```python
from build123d import *

# Parameters (mm, degrees)
SKETCH1_W              = 25.4
SKETCH1_H              = 27.78125
BOSS_EXTRUDE1_DEPTH    = 2.38125
SKETCH2_W              = 25.4
SKETCH2_H              = 2.38125
BOSS_EXTRUDE2_DEPTH    = 25.4
CONVERT_SOLID2_START   = -12.7
CONVERT_SOLID2_DEPTH   = 25.4
CONVERT_SOLID2_2_DEPTH = 25.4
FILLET1_R              = 2.54
SKETCH9_R              = 2.54
CUT_EXTRUDE1_DEPTH     = 2.38125


# Read off the part's stored shape, not the designer's step: Convert-Solid2
with BuildPart() as part:
    # Sketch1 → Boss-Extrude1 (new body)
    with BuildSketch(Plane(origin=(0, 0, 0), x_dir=(1, 0, 0), z_dir=(0, 1, 0))):
        Rectangle(SKETCH1_W, SKETCH1_H)
    extrude(amount=BOSS_EXTRUDE1_DEPTH)

    # Sketch2 → Boss-Extrude2 (add)
    with BuildSketch(Plane(origin=(0, 2.38125, 0), x_dir=(1, 0, 0), z_dir=(0, 1, 0))):
        with Locations((0, 12.7)):
            Rectangle(SKETCH2_W, SKETCH2_H)
    extrude(amount=BOSS_EXTRUDE2_DEPTH)

    # Convert-Solid2 outline → Convert-Solid2 (cut)
    with BuildSketch(Plane.YZ.offset(CONVERT_SOLID2_START)):
        with BuildLine():
            Line((0, -13.890625), (7.14375, -13.890625))
            ThreePointArc((7.14375, -13.890625), (2.092355932, -11.798269068), (0, -6.746875))
            Line((0, -6.746875), (0, -13.890625))
        make_face()
    extrude(amount=CONVERT_SOLID2_DEPTH, mode=Mode.SUBTRACT)

    # Convert-Solid2 2 outline → Convert-Solid2 2 (add)
    with BuildSketch(Plane.YZ.offset(CONVERT_SOLID2_START)):
        with BuildLine():
            Line((2.38125, -11.509375), (7.14375, -11.509375))
            ThreePointArc((7.14375, -11.509375), (3.776153955, -10.114471045), (2.38125, -6.746875))
            Line((2.38125, -6.746875), (2.38125, -11.509375))
        make_face()
    extrude(amount=CONVERT_SOLID2_2_DEPTH)

    # Fillet1
    fillet1_edges = [part.edges().sort_by_distance(p)[0] for p in [
        (-12.7, 1.190625, 13.890625),
        (12.7, 1.190625, 13.890625),
        (-12.7, 27.78125, -12.7),
        (12.7, 27.78125, -12.7),
    ]]
    fillet(fillet1_edges, radius=FILLET1_R)

    # Sketch9 → Cut-Extrude1 (cut)
    with BuildSketch(Plane(origin=(0, 2.38125, 0), x_dir=(1, 0, 0), z_dir=(0, 1, 0))):
        with Locations(Location((6.35, -7.540625, 0), (0, 0, 270))):
            Circle(SKETCH9_R)
        with Locations(Location((-6.35, -7.540625, 0), (0, 0, 270))):
            Circle(SKETCH9_R)
    extrude(amount=-CUT_EXTRUDE1_DEPTH, mode=Mode.SUBTRACT)


solid = part.part
```
Model file for the job. Use its own axes, mm. A direction names the side the tool comes from. Round coordinates to 2 decimals unless told otherwise and drop trailing zeros. Write each loop counter-clockwise with the first axis right and the second up, starting at its lowest first coordinate (ties: lowest second). Pieces come first, ordered by that corner, then holes. Notation, with made-up numbers: M 69,33 L 117,33 A16 ccw 117,43 Z; hole C -30.75,32.25 d1. An arc over 180 degrees is marked long. Put each result on its own line as item: value.
Item 1: Probe L1, parallel to Y at x = -6.75, z = 12.5; L2, parallel to Z at x = -10.75, y = 18.25; L3, parallel to Z at x = -0.25, y = 5.75. List the from-to ranges inside material, lowest first. Write a range as from..to.
Responses:
L1: 0..2.38
L2: -13.89..-11.51
L3: -13.75..-11.3
Item 2: Cut at C-C (y = 23.5). List the corners of the cut face in (x, z).
Responses:
outline: M -12.7,-13.89 L 12.7,-13.89 L 12.7,-11.51 L -12.7,-11.51 Z
Item 3: Tool access for faces 1 (the flat face through (0, 17, -11.509)), 2 (the flat face through (0, 27.781, -13)): list every direction of +Z, -Z, +X, -X, +Y, -Y with a clear straight run to the whole face (end or side of a thin tool).
Responses:
face 1: +Z, +X, -X, +Y
face 2: +Z, -Z, +X, -X, +Y
Item 4: Cut at A-A (x = 6.35). List the corners of the cut face in (y, z) (1 decimal).
Responses:
outline: M 0,-6.7 A7.1 ccw 7.1,-13.9 L 27.8,-13.9 L 27.8,-11.5 L 7.1,-11.5 A4.8 cw 2.4,-6.7 L 2.4,5 L 0,5 Z; M 0,10.1 L 2.4,10.1 L 2.4,13.9 L 0,13.9 Z
Item 5: Flat gauge pin, fed straight in: P1, Ø6, axis at x = -6.35, z = 7.54, coming from the +Y side. Where does the tip first touch, or does it go through?
Responses:
P1: y = 2.38
Item 6: Mould opens along Z. For faces 3 (the flat face through (0, 17, -13.891)), 4 (the flat face through (0, 1, 13.891)), 5 (the cylindrical face through (8.87, 1.21, 7.21)), 6 (the cylindrical face through (-8.83, 1.21, 6.99)) say: +Z half, -Z half, draft (parallel to the pull), parting line (faces both ways), or undercut.
Responses:
face 3: -Z half
face 4: +Z half
face 5: undercut
face 6: undercut
Item 7: Cut at D-D (z = -7.5). List the corners of the cut face in (x, y), and give its area (3 significant figures).
Responses:
outline: M -12.7,0.04 L 12.7,0.04 L 12.7,2.44 L -12.7,2.44 Z
area: 61.0 mm²
Item 8: Cut at B-B (z = 8.25). List the corners of the cut face in (x, y).
Responses:
outline: M -12.7,0 L -8.79,0 L -8.79,2.38 L -12.7,2.38 Z; M -3.91,0 L 3.91,0 L 3.91,2.38 L -3.91,2.38 Z; M 8.79,0 L 12.7,0 L 12.7,2.38 L 8.79,2.38 Z
